from build123d import *

# Parameters (mm, degrees)
BOSS_EXTRUDE1_DEPTH             = 20
SKETCH3_R                       = 1.975
CUT_EXTRUDE1_DEPTH              = 23.641223465
BOSS_EXTRUDE2_REACH             = 24.641
BOSS_EXTRUDE2_DIRECTION_2_REACH = 24.641
FILLET1_R                       = 1


with BuildPart() as part:
    # Sketch2 → Boss-Extrude1 (new, symmetric)
    with BuildSketch(Plane.XY):
        with BuildLine():
            Line((-1.921572875, 0), (1.921572875, 0))
            ThreePointArc((1.921572875, 0), (3.069623172, 0.228361402), (4.042893219, 0.878679656))
            Line((4.042893219, 0.878679656), (6.957106781, 3.792893219))
            ThreePointArc((6.957106781, 3.792893219), (7.173879533, 4.882683432), (6.25, 5.5))
            Line((6.25, 5.5), (3.2, 5.5))
            Line((3.2, 5.5), (3.2, 7.75))
            Line((3.2, 7.75), (-3.2, 7.75))
            Line((-3.2, 7.75), (-3.2, 5.5))
            Line((-3.2, 5.5), (-6.25, 5.5))
            ThreePointArc((-6.25, 5.5), (-7.173879533, 4.882683432), (-6.957106781, 3.792893219))
            Line((-6.957106781, 3.792893219), (-4.042893219, 0.878679656))
            ThreePointArc((-4.042893219, 0.878679656), (-3.069623172, 0.228361402), (-1.921572875, 0))
        make_face()
    extrude(amount=BOSS_EXTRUDE1_DEPTH, both=True)

    # Sketch3 → Cut-Extrude1 (cut, through all)
    with BuildSketch(Plane(origin=(0, 7.75, 0), x_dir=(1, 0, 0), z_dir=(0, 1, 0))):
        with Locations(Location((0, 15, 0), (0, 0, 270))):
            Circle(SKETCH3_R)
        with Locations(Location((0, -15, 0), (0, 0, 346.642693005))):
            Circle(SKETCH3_R)
    extrude(amount=-CUT_EXTRUDE1_DEPTH, mode=Mode.SUBTRACT)

    # Boss-Extrude2: up to this face of the body (flat: up to its plane)
    boss_extrude2_end = Plane(part.part.faces().sort_by_distance((3.2, 6.625, 0))[0])
    # Sketch4 → Boss-Extrude2 (add, up to the picked face)
    with BuildSketch(Plane(origin=(0, 0, 0), x_dir=(0, 0, -1), z_dir=(1, 0, 0)), mode=Mode.PRIVATE) as boss_extrude2_sk1:
        Polygon((-10, 17.75), (-10, 7.75), (0, 7.75), align=None)
    boss_extrude2_tool1 = split(extrude(boss_extrude2_sk1.sketch, amount=BOSS_EXTRUDE2_REACH, mode=Mode.PRIVATE), bisect_by=boss_extrude2_end, keep=Keep.BOTH, mode=Mode.PRIVATE)
    # Sketch4 → Boss-Extrude2 (add, up to the picked face)
    with BuildSketch(Plane(origin=(0, 0, 0), x_dir=(0, 0, -1), z_dir=(1, 0, 0)), mode=Mode.PRIVATE) as boss_extrude2_sk2:
        Polygon((10, 17.75), (0, 7.75), (10, 7.75), align=None)
    boss_extrude2_tool2 = split(extrude(boss_extrude2_sk2.sketch, amount=BOSS_EXTRUDE2_REACH, mode=Mode.PRIVATE), bisect_by=boss_extrude2_end, keep=Keep.BOTH, mode=Mode.PRIVATE)
    add(boss_extrude2_tool1.solids().sort_by(Axis((0, 11.083333, 6.666667), (1, 0, 0)))[0])
    add(boss_extrude2_tool2.solids().sort_by(Axis((0, 11.083333, -6.666667), (1, 0, 0)))[0])

    # Boss-Extrude2 direction 2: up to this face of the body (flat: up to its plane)
    boss_extrude2_direction_2_end = Plane(part.part.faces().sort_by_distance((-3.2, 6.625, 0))[0])
    # Sketch4 → Boss-Extrude2 direction 2 (add, up to the picked face)
    with BuildSketch(Plane(origin=(0, 0, 0), x_dir=(0, 0, -1), z_dir=(1, 0, 0)), mode=Mode.PRIVATE) as boss_extrude2_direction_2_sk1:
        Polygon((-10, 17.75), (-10, 7.75), (0, 7.75), align=None)
    boss_extrude2_direction_2_tool1 = split(extrude(boss_extrude2_direction_2_sk1.sketch, amount=-BOSS_EXTRUDE2_DIRECTION_2_REACH, mode=Mode.PRIVATE), bisect_by=boss_extrude2_direction_2_end, keep=Keep.BOTH, mode=Mode.PRIVATE)
    # Sketch4 → Boss-Extrude2 direction 2 (add, up to the picked face)
    with BuildSketch(Plane(origin=(0, 0, 0), x_dir=(0, 0, -1), z_dir=(1, 0, 0)), mode=Mode.PRIVATE) as boss_extrude2_direction_2_sk2:
        Polygon((10, 17.75), (0, 7.75), (10, 7.75), align=None)
    boss_extrude2_direction_2_tool2 = split(extrude(boss_extrude2_direction_2_sk2.sketch, amount=-BOSS_EXTRUDE2_DIRECTION_2_REACH, mode=Mode.PRIVATE), bisect_by=boss_extrude2_direction_2_end, keep=Keep.BOTH, mode=Mode.PRIVATE)
    add(boss_extrude2_direction_2_tool1.solids().sort_by(Axis((0, 11.083333, 6.666667), (-1, 0, 0)))[0])
    add(boss_extrude2_direction_2_tool2.solids().sort_by(Axis((0, 11.083333, -6.666667), (-1, 0, 0)))[0])

    # Fillet1
    fillet1_edges = [part.edges().sort_by_distance(p)[0] for p in [
        (0, 17.75, 10),
        (0, 7.75, 0),
        (0, 17.75, -10),
    ]]
    fillet(fillet1_edges, radius=FILLET1_R)


solid = part.part
Geometry: final body of the model. Coordinates: model frame, mm. A direction names the side the tool comes from. Coordinates: 2 decimals unless noted, no trailing zeros. Order: outer loops, then holes, each group sorted by start corner. A loop starts at its lowest first (then second) coordinate and runs counter-clockwise, first axis right, second up.
(1) Section query D-D (y = 6.75). Return the cut outline in (x, z) (3 decimals), plus the area to 3 significant figures.
(2) Draft query along X for faces 1 (the face through (3.2, 7, 0)), 2 (the face through (0.593, 3.929, -13.116)), 3 (the face through (0, 4, -20)). Return one class per face: pulls with the +X half, pulls with the -X half, needs draft (parallel to the pull), parting line crosses it, or undercut.
(3) Section query C-C (z = -15). Return the cut outline in (x, y) (3 decimals), plus the area to 3 significant figures.
(4) Section query B-B (z = 3.5). Return the cut outline in (x, y).
(5) First-contact query: pin 1 (5 mm diameter, centred on x = 0, z = 14, fed in from +Y); pin 2 (3.5 mm diameter, centred on y = 9.5, z = -7, fed in from +X); pin 3 (5 mm diameter, centred on x = -1, y = 11, fed in from +Z). Flat tips, straight axial feed; report the tip coordinate or a pass-through.
(6) Section query A-A (x = 0). Return the cut outline in (y, z) (3 decimals), plus the area to 3 significant figures.
(7) Material intervals for probe 1 along Z at (x, y) = (0, 4.75) (3 decimals); probe 2 along X at (y, z) = (4.5, -15) (3 decimals); probe 3 along X at (y, z) = (6.25, -15) (3 decimals), sorted ascending.
(8) Access query for faces 4 (the face through (2.2, 7.75, -14.9)), 5 (the face through (5, 5.5, 0)), 6 (the face through (2.2, 7.75, 15.1)), 7 (the face through (-5, 5.5, 0)), 8 (the face through (0.04, 12.3, -4.55)). Directions: +Z, -Z, +X, -X, +Y, -Y. A direction counts if a zero-diameter tool reaches every point of the face in a straight line with its end or side. Return the directions, or none.
Solution:
1. outline: (-3.2, -20) - (3.2, -20) - (3.2, 20) - (-3.2, 20) - close; hole circle Ø3.95 at (0, -15); hole circle Ø3.95 at (0, 15)
1. area: 231 mm2
2. face 1: pulls with the +X half
2. face 2: undercut
2. face 3: needs draft
3. outline: (-6.957, 3.793) - (-4.043, 0.879) arc R3 ccw to (-1.975, 0) - (-1.975, 7.75) - (-3.2, 7.75) - (-3.2, 5.5) - (-6.25, 5.5) arc R1 ccw to start; (1.975, 0) arc R3 ccw to (4.043, 0.879) - (6.957, 3.793) arc R1 ccw to (6.25, 5.5) - (3.2, 5.5) - (3.2, 7.75) - (1.975, 7.75) - close
3. area: 46.0 mm2
4. outline: (-6.96, 3.79) - (-4.04, 0.88) arc R3 ccw to (-1.92, 0) - (1.92, 0) arc R3 ccw to (4.04, 0.88) - (6.96, 3.79) arc R1 ccw to (6.25, 5.5) - (3.2, 5.5) - (3.2, 11.25) - (-3.2, 11.25) - (-3.2, 5.5) - (-6.25, 5.5) arc R1 ccw to start
5. pin 1: stops at y = 7.75
5. pin 2: stops at x = 3.2
5. pin 3: stops at z = 10
6. outline: (0, -20) - (7.75, -20) - (7.75, -16.975) - (0, -16.975) - close; (0, -13.025) - (7.75, -13.025) - (7.75, -10) - (15.336, -10) arc R1 ccw to (16.043, -8.293) - (8.457, -0.707) arc R1 cw to (8.457, 0.707) - (16.043, 8.293) arc R1 ccw to (15.336, 10) - (7.75, 10) - (7.75, 13.025) - (0, 13.025) - close; (0, 16.975) - (7.75, 16.975) - (7.75, 20) - (0, 20) - close
6. area: 347 mm2
7. probe 1: z = -20 to -16.975, -13.025 to 13.025, 16.975 to 20
7. probe 2: x = -7.25 to -1.975, 1.975 to 7.25
7. probe 3: x = -3.2 to -1.975, 1.975 to 3.2
8. face 4: -Z, +X, -X, +Y
8. face 5: +Z, -Z, +X, +Y
8. face 6: +Z, +X, -X, +Y
8. face 7: +Z, -Z, -X, +Y
8. face 8: +X, -X, +Y
